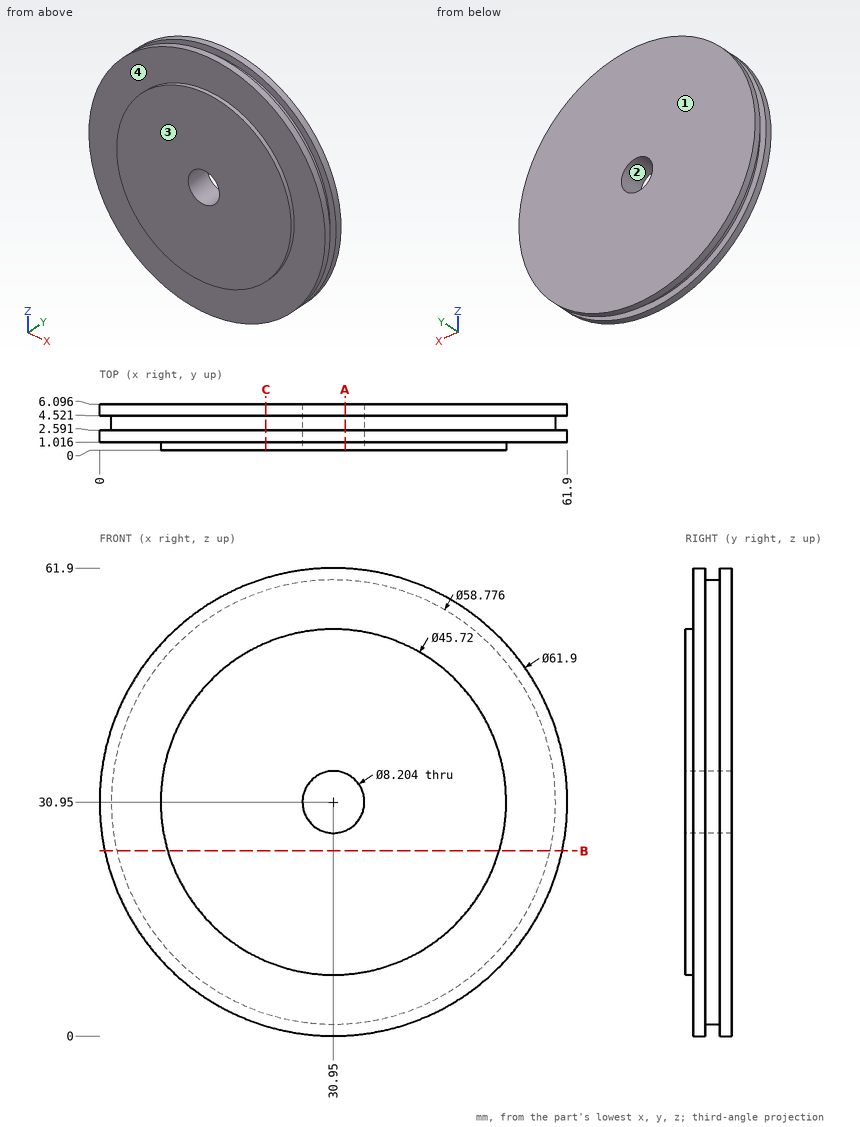
Geometry: see drawing. Coordinates: mm, zero at the bounding-box minimum. A direction names the side the tool comes from. Round coordinates to 2 decimals unless told otherwise and drop trailing zeros. Loops run counter-clockwise (first coordinate to the right, second up) from the corner with the lowest first, then second, coordinate; pieces in that order, holes last. Notation, with made-up numbers: (-22, -6.75) -> (31, -6.75) arc R14 ccw to (31, 7.25) -> close; hole circle Ø11 at (69, -3.5). An arc over 180 degrees is marked (long way). Write each question's results on one line, items separated by ' | '.
Item 1: Cut plane A-A on x = 32.5. Return the cut outline in (y, z), and give its area (3 significant figures).
Answers below:
outline: (0, 8.14) -> (1.02, 8.14) -> (1.02, 0.04) -> (2.59, 0.04) -> (2.59, 1.6) -> (4.52, 1.6) -> (4.52, 0.04) -> (6.1, 0.04) -> (6.1, 27.15) -> (0, 27.15) -> close; (0, 34.75) -> (6.1, 34.75) -> (6.1, 61.86) -> (4.52, 61.86) -> (4.52, 60.3) -> (2.59, 60.3) -> (2.59, 61.86) -> (1.02, 61.86) -> (1.02, 53.76) -> (0, 53.76) -> close | area: 308 mm²
Item 2: Pin query (flat end, axial travel): pin 1 Ø6.5 at (x, z) = (30.95, 30.95) entering from +Y; pin 2 Ø3 at (y, z) = (4.5, 50.5) entering from -X; pin 3 Ø1.5 at (y, z) = (3.5, 55.5) entering from +X. Return the tip coordinate at first contact, or that it passes through.
Answers below:
pin 1: passes through | pin 2: stops at x = 5.81 | pin 3: stops at x = 48.19
Item 3: Set-up query: the marked faces 3 and 4. Return all of +Z, -Z, +X, -X, +Y, -Y with unobstructed straight access to the full face (end or side cutting, diameter ignored); none if empty.
Answers below:
face 3: +Z, -Z, +X, -X, -Y | face 4: -Y
Item 4: Line query: probe 1 along Y at (x, z) = (55.5, 14); probe 2 along Y at (x, z) = (20.5, 9); probe 3 along X at (y, z) = (5.5, 31.5) (1 decimal). Output: solid intervals per line, ascending. Write a range as [from, to].
Answers below:
probe 1: y = [1.02, 2.59], [4.52, 6.1] | probe 2: y = [1.02, 6.1] | probe 3: x = [0, 26.9], [35, 61.9]
Item 5: Cut plane B-B on z = 24.5. Return the cut outline in (x, y).
Answers below:
outline: (0.68, 1.02) -> (9.02, 1.02) -> (9.02, 0) -> (52.88, 0) -> (52.88, 1.02) -> (61.22, 1.02) -> (61.22, 2.59) -> (59.62, 2.59) -> (59.62, 4.52) -> (61.22, 4.52) -> (61.22, 6.1) -> (0.68, 6.1) -> (0.68, 4.52) -> (2.28, 4.52) -> (2.28, 2.59) -> (0.68, 2.59) -> close
Item 6: Cut plane C-C on x = 22. Return the cut outline in (y, z) (1 decimal).
Answers below:
outline: (0, 9.9) -> (1, 9.9) -> (1, 1.3) -> (2.6, 1.3) -> (2.6, 3) -> (4.5, 3) -> (4.5, 1.3) -> (6.1, 1.3) -> (6.1, 60.6) -> (4.5, 60.6) -> (4.5, 58.9) -> (2.6, 58.9) -> (2.6, 60.6) -> (1, 60.6) -> (1, 52) -> (0, 52) -> close
Item 7: Pull-direction query (X, two-part tool) for the marked faces 1 and 2; classes: pulls with the +X half, pulls with the -X half, needs draft (parallel to the pull), parting line crosses it, or undercut.
Answers below:
face 1: needs draft | face 2: undercut
